The model under review builds one solid part; all positions refer to its coordinate system, in mm. Face numbers are marked on the shaded views. A direction names the side the tool comes from. Coordinates: 2 decimals unless noted, no trailing zeros. Loops run counter-clockwise (first coordinate to the right, second up) from the corner with the lowest first, then second, coordinate; pieces in that order, holes last. Notation, with made-up numbers: (-23, 83) - (23, 83) arc R11 cw to (23, 97) - close; hole circle Ø5 at (9.25, -24). An arc over 180 degrees is marked (long way). Answer in a Markdown table with one row per item. Add a question column.
(1) Machinability: for the marked faces 4, 5 and 6, which of the approach directions +Z, -Z, +X, -X, +Y, -Y give a long, thin tool a straight path to every point of the face, cutting with its end or side? Answer none if there is none.
(2) We need section A-A on y = 0. Write out the cut boundary in (x, z), plus the area to 3 significant figures.
(3) For line 1 along Z through (x, y) = (1.1, -1.5); line 2 along X through (y, z) = (0.7, 2.75); line 3 along Z through (x, y) = (0.3, 1.8), list the stretches that pass through material, from the lowest coordinate up.
(4) We need section B-B on x = 0. Write out the cut boundary in (y, z), plus the area to 3 significant figures.
(5) Mouldability with a two-part tool opening along X and no side actions: class the marked faces 1, 2 and 3 as +X half, -X half, draft (parallel to the pull), parting line (faces both ways), or undercut.
(6) We need section C-C on z = 1. Write out the cut boundary in (x, y).
(7) For P1, Ø0.8, axis at x = 0, y = 0, coming from the +Z side; P2, Ø2, axis at x = 1, z = -0.5, coming from the +Y side, all flat-tipped, find the tip position at first contact; note any pin that passes through.
(8) We need section D-D on y = 1.5. Write out the cut boundary in (x, z), plus the area to 3 significant figures.
from build123d import *

# Parameters (mm, degrees)
ESQUISSE1_R                     = 2
BASE_EXTRUSION_DEPTH            = 3
ESQUISSE2_R                     = 1
BOSS_EXTRU_1_DEPTH              = 4
CHANFREIN2_SIZE                 = 2.5
CHANFREIN2_SIZE2                = 0.440817452
ESQUISSE3_W                     = 1
ESQUISSE3_H                     = 4.690148878
ENL_V_DE_MAT_EXTRU_MINCE1_DEPTH = 1.5


with BuildPart() as part:
    # Esquisse1 → Base-Extrusion (new body)
    with BuildSketch(Plane.XY):
        Circle(ESQUISSE1_R)
    extrude(amount=BASE_EXTRUSION_DEPTH)

    # Esquisse2 → Boss.-Extru.1 (add)
    with BuildSketch(Plane(origin=(0, 0, 0), x_dir=(-1, 0, 0), z_dir=(0, 0, -1))):
        with Locations(Location((0, 0, 0), (0, 0, 180))):
            Circle(ESQUISSE2_R)
    extrude(amount=BOSS_EXTRU_1_DEPTH)

    # Chanfrein2
    chanfrein2_edges = [part.edges().sort_by_distance(p)[0] for p in [
        (-1, 0, -4),
    ]]
    chanfrein2_side = [part.faces().sort_by_distance(p)[0] for p in [
        (-1, 0, -2),
    ]]
    chamfer(chanfrein2_edges, length=CHANFREIN2_SIZE, length2=CHANFREIN2_SIZE2, reference=chanfrein2_side[0])

    # Esquisse3 → Enlèv. de mat.-Extru.-Mince1 (cut)
    with BuildSketch(Plane.XY.offset(3)):
        with Locations((0, -0.083649642)):
            Rectangle(ESQUISSE3_W, ESQUISSE3_H)
    extrude(amount=-ENL_V_DE_MAT_EXTRU_MINCE1_DEPTH, mode=Mode.SUBTRACT)


solid = part.part
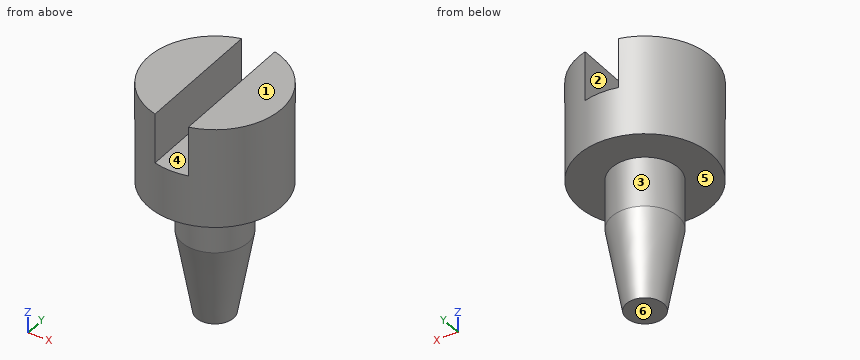
Outcome:
| question | item | result |
|---|---|---|
| 1 | face 4 | +Z, +Y, -Y |
| 1 | face 5 | -Z |
| 1 | face 6 | -Z, +X, -X, +Y, -Y |
| 2 | outline | (-2, 0) - (-1, 0) - (-1, -1.5) - (-0.56, -4) - (0.56, -4) - (1, -1.5) - (1, 0) - (2, 0) - (2, 3) - (0.5, 3) - (0.5, 1.5) - (-0.5, 1.5) - (-0.5, 3) - (-2, 3) - close |
| 2 | area | 17.4 mm² |
| 3 | line 1 | 0 to 3 |
| 3 | line 2 | -1.87 to -0.5, 0.5 to 1.87 |
| 3 | line 3 | 0 to 1.5 |
| 4 | outline | (-2, 0) - (-1, 0) - (-1, -1.5) - (-0.56, -4) - (0.56, -4) - (1, -1.5) - (1, 0) - (2, 0) - (2, 1.5) - (-2, 1.5) - close |
| 4 | area | 12.9 mm² |
| 5 | face 1 | draft |
| 5 | face 2 | undercut |
| 5 | face 3 | parting line |
| 6 | outline | circle Ø4 at (0, 0) |
| 7 | P1 | z = 1.5 |
| 7 | P2 | y = 2 |
| 8 | outline | (-1.32, 0) - (1.32, 0) - (1.32, 3) - (0.5, 3) - (0.5, 1.5) - (-0.5, 1.5) - (-0.5, 3) - (-1.32, 3) - close |
| 8 | area | 6.44 mm² |
